The model under review builds one solid part; all positions refer to its coordinate system, in mm. A direction names the side the tool comes from. Coordinates: 2 decimals unless noted, no trailing zeros. Loops run counter-clockwise (first coordinate to the right, second up) from the corner with the lowest first, then second, coordinate; pieces in that order, holes last. Notation, with made-up numbers: M 58.5,87 L 94.5,87 A17 cw 94.5,91 Z; hole C 2,-17 d3. An arc over 180 degrees is marked long. Write item = value, one per line. Start each with the question number.
Q1. Mouldability with a two-part tool opening along X and no side actions: class faces 5 (the face through (0, 0, 0)), 6 (the face through (-26.121, -8.487, 4.93)), 7 (the face through (-7.89, 25.17, 4.93)), 8 (the face through (21.5, 15.28, 4.93)) as released by +X, released by -X, zero draft, split by the parting line, or undercut.
Q2. We need section C-C on y = 12.5. Give the boundary of the cut face in (x, z).
Q3. For faces 1 (the face through (-16.144, -22.22, 4.93)), 2 (the face through (0, -27, 5)), 3 (the face through (26.121, 8.487, 4.93)), 4 (the face through (16.144, -22.22, 4.93)), list the 3-axis set-ups (+Z, -Z, +X, -X, +Y, -Y) from which the entire face can be reached by the end or side of a thin tool; tool diameter is ignored.
Q4. Clearance check with flat-ended pins moving along their axes: pin 1 Ø4 at (y, z) = (-28.5, 3) entering from -X; pin 2 Ø8 at (x, y) = (18, -1) entering from +Z; pin 3 Ø8 at (x, z) = (9, 6) entering from +Y. State where each tip first meets the part, or that it passes through.
Q5. We need section B-B on x = -5. Give the boundary of the cut face in (y, z).
Q6. Wall thickness on probe 1 along Y at (x, z) = (-1.5, 22); probe 2 along Z at (x, y) = (-10, -1.5); probe 3 along Y at (x, z) = (-17, 7): over which ranges is each line inside the solid? List them lowest first.
Q7. We need section D-D on x = 22. Give the boundary of the cut face in (y, z), and give its area (3 significant figures).
from build123d import *

# Parameters (mm, degrees)
F1_DEPTH = 10
F2_R     = 4.167492
F3_DEPTH = 25
F4_R     = 1.638952
F5_DEPTH = 25
F6_R     = 1.638952
F7_DEPTH = 47.6


with BuildPart() as f1:
    # F0 (on Top) → F1 (new body)
    with BuildSketch(Plane.XY):
        with BuildLine():
            Line((0, 25), (0, 30))
            ThreePointArc((0, 30), (-0.639446, 29.993184), (-1.278602, 29.972741))
            Line((-1.278602, 29.972741), (-14.694631, 20.225425))
            Line((-14.694631, 20.225425), (-17.633558, 24.27051))
            ThreePointArc((-17.633558, 24.27051), (-18.146874, 23.889139), (-18.651946, 23.496913))
            Line((-18.651946, 23.496913), (-23.776413, 7.725425))
            Line((-23.776413, 7.725425), (-28.531695, 9.27051))
            ThreePointArc((-28.531695, 9.27051), (-28.722813, 8.660254), (-28.90088, 8.046063))
            Line((-28.90088, 8.046063), (-23.776413, -7.725425))
            Line((-23.776413, -7.725425), (-28.531695, -9.27051))
            ThreePointArc((-28.531695, -9.27051), (-28.327614, -9.876553), (-28.11066, -10.478109))
            Line((-28.11066, -10.478109), (-14.694631, -20.225425))
            Line((-14.694631, -20.225425), (-17.633558, -24.27051))
            ThreePointArc((-17.633558, -24.27051), (-17.112228, -24.640853), (-16.583124, -25))
            Line((-16.583124, -25), (0, -25))
            Line((0, -25), (0, -30))
            ThreePointArc((0, -30), (0.639446, -29.993184), (1.278602, -29.972741))
            Line((1.278602, -29.972741), (14.694631, -20.225425))
            Line((14.694631, -20.225425), (17.633558, -24.27051))
            ThreePointArc((17.633558, -24.27051), (18.146874, -23.889139), (18.651946, -23.496913))
            Line((18.651946, -23.496913), (23.776413, -7.725425))
            Line((23.776413, -7.725425), (28.531695, -9.27051))
            ThreePointArc((28.531695, -9.27051), (28.722813, -8.660254), (28.90088, -8.046063))
            Line((28.90088, -8.046063), (23.776413, 7.725425))
            Line((23.776413, 7.725425), (28.531695, 9.27051))
            ThreePointArc((28.531695, 9.27051), (28.327614, 9.876553), (28.11066, 10.478109))
            Line((28.11066, 10.478109), (14.694631, 20.225425))
            Line((14.694631, 20.225425), (17.633558, 24.27051))
            ThreePointArc((17.633558, 24.27051), (17.112228, 24.640853), (16.583124, 25))
            Line((16.583124, 25), (0, 25))
        make_face()
    extrude(amount=F1_DEPTH)

    # F2 (on face) → F3 (join)
    with BuildSketch(Plane.XY.offset(10)):
        with Locations((-1.638952, -5.852238)):
            Circle(F2_R)
    extrude(amount=F3_DEPTH)

    # F4 (on face) → F5 (cut)
    with BuildSketch(Plane.XY.offset(10)):
        with Locations((-1.638952, -5.852238)):
            Circle(F4_R)
    extrude(amount=-F5_DEPTH, mode=Mode.SUBTRACT)

    # F6 (on face) → F7 (cut)
    with BuildSketch(Plane.XY.offset(10)):
        with Locations((-1.638952, -5.852238)):
            Circle(F6_R)
    extrude(amount=F7_DEPTH, mode=Mode.SUBTRACT)


solid = f1.part
Returned:
q1.face_5 = zero draft
q1.face_6 = released by -X
q1.face_7 = undercut
q1.face_8 = released by +X
q2.outline = M -22.23,0 L 25.33,0 L 25.33,10 L -22.23,10 Z
q3.face_1 = +Z, -Z, -X
q3.face_2 = +Z, -Z, -X, -Y
q3.face_3 = +Z, -Z, +X
q3.face_4 = +Z, -Z, -Y
q4.pin_1 = 0
q4.pin_2 = 10
q4.pin_3 = 25
q5.outline = M -25,0 L 27.27,0 L 27.27,10 L -3.39,10 L -3.39,35 L -8.32,35 L -8.32,10 L -25,10 Z
q6.probe_1 = -10.02 to -7.49, -4.22 to -1.69
q6.probe_2 = 0 to 10
q6.probe_3 = -24.72 to -23.4, -18.55 to 23.4
q7.outline = M -13.19,0 L 14.92,0 L 14.92,10 L -13.19,10 Z
q7.area = 281 mm^2
